CAD build for the part. Positions are in the model's coordinates, mm. A direction names the side the tool comes from. Round coordinates to 2 decimals unless told otherwise and drop trailing zeros. Order: outer loops, then holes, each group sorted by start corner. A loop starts at its lowest first (then second) coordinate and runs counter-clockwise, first axis right, second up. Notation, with made-up numbers: M 31,56.5 L 35,56.5 A24 ccw 35,81.5 Z; hole C -4.75,6.5 d9. An arc over 180 degrees is marked long. Answer as a JSON object with one key per item and string values.
```python
from build123d import *

# Parameters (mm, degrees)
BOSS_EXTRUDE1_DEPTH = 15
SKETCH3_R           = 2.65
CUT_EXTRUDE1_DEPTH  = 15
M3_TAPPED_HOLE1_D   = 2.5
SKETCH7_R           = 4
CUT_EXTRUDE2_DEPTH  = 2


with BuildPart() as part:
    # Sketch1 → Boss-Extrude1 (new body)
    with BuildSketch(Plane.XY):
        Polygon((35, 0), (17, 0), (17, 3), (0, 3), (0, 25), (10, 25), (10, 12), (35, 12), align=None)
    extrude(amount=BOSS_EXTRUDE1_DEPTH)

    # Sketch3 → Cut-Extrude1 (cut)
    with BuildSketch(Plane(origin=(10, 0, 0), x_dir=(0, 0, -1), z_dir=(1, 0, 0))):
        with Locations((-7.5, 18.5)):
            Circle(SKETCH3_R)
    extrude(amount=-CUT_EXTRUDE1_DEPTH, mode=Mode.SUBTRACT)

    # M3 Tapped Hole1 (through all)
    with Locations(Plane(origin=(25, 6, 15), x_dir=(1, 0, 0), z_dir=(0, 0, 1))):
        with Locations((0, 0)):
            Hole(M3_TAPPED_HOLE1_D / 2)

    # Sketch7 → Cut-Extrude2 (cut)
    with BuildSketch(Plane.XY.offset(15)):
        with Locations((25, 6)):
            Circle(SKETCH7_R)
    extrude(amount=-CUT_EXTRUDE2_DEPTH, mode=Mode.SUBTRACT)


solid = part.part
```
Item 1: Saw through at D-D on z = 1.5. List the corners of the cut face in (x, y).
Worked answers:
{"outline": "M 0,3 L 17,3 L 17,0 L 35,0 L 35,12 L 10,12 L 10,25 L 0,25 Z; hole C 25,6 d2.5"}
Item 2: Wall check: line 1 along Y through (x, z) = (25, 13.9); line 2 along Y through (x, z) = (5.75, 7.5); line 3 along X through (y, z) = (5, 1). Give the ranges that are in metal, low to high. Write a range as [from, to].
Worked answers:
{"line 1": "y = [0, 2], [10, 12]", "line 2": "y = [3, 15.85], [21.15, 25]", "line 3": "x = [0, 24.25], [25.75, 35]"}
Item 3: Saw through at A-A on z = 7.5. List the corners of the cut face in (x, y).
Worked answers:
{"outline": "M 0,3 L 17,3 L 17,0 L 35,0 L 35,12 L 10,12 L 10,15.85 L 0,15.85 Z; M 0,21.15 L 10,21.15 L 10,25 L 0,25 Z; hole C 25,6 d2.5"}
Item 4: 3-axis set-ups, long thin cutter, end or side, ignore diameter. For faces 5 (the flat face through (14, 10, 15)), 6 (the cylindrical face through (21.8, 3.6, 14)), 7 (the flat face through (17, 1, 7)): which of +Z, -Z, +X, -X, +Y, -Y reach the whole face in a straight line?
Worked answers:
{"face 5": "+Z, +X, -X, +Y, -Y", "face 6": "+Z", "face 7": "+Z, -Z, -X, -Y"}
Item 5: Two-plate mould, pull along X, no slides. Class faces 1 (the flat face through (10, 21.5, 7.4)), 2 (the flat face through (26, 7, 13)), 3 (the flat face through (0, 14, 7)), 4 (the flat face through (22, 12, 7)): released by +X, released by -X, zero draft, split by the parting line, or undercut.
Worked answers:
{"face 1": "released by +X", "face 2": "undercut", "face 3": "released by -X", "face 4": "zero draft"}
Item 6: Saw through at B-B on y = 20.75. List the corners of the cut face in (x, z).
Worked answers:
{"outline": "M 0,0 L 10,0 L 10,6.1 L 0,6.1 Z; M 0,8.9 L 10,8.9 L 10,15 L 0,15 Z"}
Item 7: Saw through at C-C on x = 25. List the corners of the cut face in (y, z), and give its area (4 significant figures).
Worked answers:
{"outline": "M 0,0 L 4.75,0 L 4.75,13 L 2,13 L 2,15 L 0,15 Z; M 7.25,0 L 12,0 L 12,15 L 10,15 L 10,13 L 7.25,13 Z", "area": "131.5 mm2"}
Item 8: Drop flat-ended pins along their axis: pin 1 Ø3 at (y, z) = (22, 9.5) entering from +X; pin 2 Ø0.9 at (y, z) = (1.5, 7) entering from -X; pin 3 Ø7.5 at (x, z) = (4.5, 8) entering from -Y. Give the stop position or say it passes through.
Worked answers:
{"pin 1": "stops at x = 10", "pin 2": "stops at x = 17", "pin 3": "stops at y = 3"}
